Verification items for the finished model (mm, model axes). Face numbers are marked on the shaded views. A direction names the side the tool comes from. Round coordinates to 2 decimals unless told otherwise and drop trailing zeros. Order: outer loops, then holes, each group sorted by start corner. A loop starts at its lowest first (then second) coordinate and runs counter-clockwise, first axis right, second up. Notation, with made-up numbers: (-29.5, 17) -> (-15.5, 17) arc R15 ccw to (-15.5, 41) -> close; hole circle Ø3 at (20, 69.25). An arc over 180 degrees is marked (long way). Return JSON: item names as keys, results as strings. Group by question number.
Item 1: Sectioned sample at B-B on z = 0.3. Give the number of separate pieces and of enclosed holes in the cut face, plus the area to 3 significant figures.
Item 2: Scan lines: probe 1 along X at (y, z) = (-0.75, 0.05); probe 2 along X at (y, z) = (-3, 1.25); probe 3 along Z at (x, y) = (-2, -4.5). Record each from-to range of solid material in increasing order. Write a range as from..to.
Item 3: Draft check along X on the marked faces 4 and 5. Enter one of: pulls with the +X half, pulls with the -X half, needs draft (parallel to the pull), parting line crosses it, or undercut.
Item 4: Access from +Z, -Z, +X, -X, +Y, -Y to the whole of each face (thin tool, end or side, straight path). Record for the marked faces 1, 2 and 3.
Item 5: Depth check by flat-ended pin: pin 1 Ø1 at (y, z) = (1, 1) entering from +X; pin 2 Ø3 at (x, y) = (-9.5, 3) entering from +Z. Enter the tip coordinate at first touch or a pass-through.
Item 6: Sectioned sample at D-D on y = -3.25. Record the cut outline in (x, z).
Item 7: Sectioned sample at C-C on x = -4.5. Record the cut outline in (y, z).
Item 8: Sectioned sample at A-A on y = -0.25. Record the cut outline in (x, z).
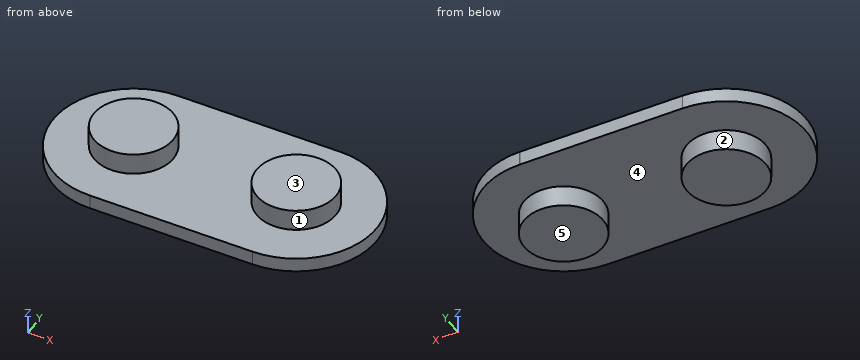
```python
from build123d import *

# Parameters (mm, degrees)
F0_R     = 1.016
F1_DEPTH = 1.016
F2_R     = 2.794
F3_DEPTH = 1.524
F4_R     = 2.794
F5_DEPTH = 1.524


with BuildPart() as f1:
    # F0 (on Top) → F1 (new body)
    with BuildSketch(Plane.XY):
        with BuildLine():
            Line((-7.064182, -6.594037), (4.492818, -6.594037))
            ThreePointArc((4.492818, -6.594037), (10.144311, -0.951402), (4.510547, 4.708935))
            ThreePointArc((4.510547, 4.708935), (4.492832, 4.708963), (4.475116, 4.708935))
            Line((4.475116, 4.708935), (-7.064182, 4.708963))
            ThreePointArc((-7.064182, 4.708963), (-12.715682, -0.942537), (-7.064182, -6.594037))
        make_face()
        with Locations((-7.064182, -0.942537)):
            Circle(F0_R, mode=Mode.SUBTRACT)
        with Locations((4.492818, -0.942537)):
            Circle(F0_R, mode=Mode.SUBTRACT)
    extrude(amount=F1_DEPTH)

    # F2 (on face) → F3 (join)
    with BuildSketch(Plane.XY.offset(1.016)):
        with Locations((4.492818, -0.942537)):
            Circle(F2_R)
        with Locations((-7.064182, -0.942537)):
            Circle(F2_R)
    extrude(amount=F3_DEPTH)

    # F4 (on face) → F5 (join)
    with BuildSketch(Plane(origin=(0, 0, 0), x_dir=(1, 0, 0), z_dir=(0, 0, -1))):
        with Locations((4.492818, 0.942537)):
            Circle(F4_R)
        with Locations((-7.064182, 0.942537)):
            Circle(F4_R)
    extrude(amount=F5_DEPTH)


solid = f1.part
```
Recorded:
{
 "1": {"separate pieces": "1", "enclosed holes": "2", "area": "224 mm²"},
 "2": {"probe 1": "-12.71..-8.06, -6.07..3.5, 5.49..10.14", "probe 2": "-8.95..-5.17, 2.6..6.38", "probe 3": "0..1.02"},
 "3": {"face 4": "undercut", "face 5": "needs draft"},
 "4": {"face 1": "+Z", "face 2": "-Z", "face 3": "+Z, +X, -X, +Y, -Y"},
 "5": {"pin 1": "x = 9.96", "pin 2": "z = 1.02"},
 "6": {"outline": "(-12.22, 0) -> (-8.64, 0) -> (-8.64, -1.52) -> (-5.49, -1.52) -> (-5.49, 0) -> (2.92, 0) -> (2.92, -1.52) -> (6.07, -1.52) -> (6.07, 0) -> (9.65, 0) -> (9.65, 1.02) -> (6.07, 1.02) -> (6.07, 2.54) -> (2.92, 2.54) -> (2.92, 1.02) -> (-5.49, 1.02) -> (-5.49, 2.54) -> (-8.64, 2.54) -> (-8.64, 1.02) -> (-12.22, 1.02) -> close"},
 "7": {"outline": "(-6.59, 0) -> (-2.05, 0) -> (-2.05, -1.52) -> (0.17, -1.52) -> (0.17, 0) -> (4.71, 0) -> (4.71, 1.02) -> (0.17, 1.02) -> (0.17, 2.54) -> (-2.05, 2.54) -> (-2.05, 1.02) -> (-6.59, 1.02) -> close"},
 "8": {"outline": "(-12.67, 0) -> (-9.77, 0) -> (-9.77, -1.52) -> (-4.36, -1.52) -> (-4.36, 0) -> (1.79, 0) -> (1.79, -1.52) -> (7.2, -1.52) -> (7.2, 0) -> (10.1, 0) -> (10.1, 1.02) -> (7.2, 1.02) -> (7.2, 2.54) -> (1.79, 2.54) -> (1.79, 1.02) -> (-4.36, 1.02) -> (-4.36, 2.54) -> (-9.77, 2.54) -> (-9.77, 1.02) -> (-12.67, 1.02) -> close; hole (-7.81, 0) -> (-6.32, 0) -> (-6.32, 1.02) -> (-7.81, 1.02) -> close; hole (3.75, 0) -> (5.24, 0) -> (5.24, 1.02) -> (3.75, 1.02) -> close"}
}
